```python
from build123d import *

# Parameters (mm, degrees)
F1_DEPTH = 38.1
F2_SIZE  = 8.763


with BuildPart() as f1:
    # F0 (on Front) → F1 (new body)
    with BuildSketch(Plane.XZ):
        Polygon((-6.977107, 9.66563), (-12.7, 0), (-8.651809, -10.447565), (4.802615, -10.447565), (10.988482, 0), (7.243273, 9.66563), align=None)
    extrude(amount=F1_DEPTH)

    # F2
    f2_edges = [f1.edges().sort_by_distance(p)[0] for p in [
        (0.133083, 0, 9.66563),
        (-9.838553, 0, 4.832815),
        (-10.675905, 0, -5.223783),
        (-1.924597, 0, -10.447565),
        (7.895549, 0, -5.223783),
        (9.115878, 0, 4.832815),
    ]]
    chamfer(f2_edges, length=F2_SIZE)


solid = f1.part
```
The listing builds one solid part. Answer for the finished solid, in the listing's coordinates (mm). Coordinates: 2 decimals unless noted, no trailing zeros. Write each loop counter-clockwise with the first axis right and the second up, starting at its lowest first coordinate (ties: lowest second). Pieces come first, ordered by that corner, then holes.
Q1. Section A-A, the plane y = -24 is taken. Write down the section's boundary in (x, z).
Returned:
outline: (-12.7, 0) - (-8.65, -10.45) - (4.8, -10.45) - (10.99, 0) - (7.24, 9.67) - (-6.98, 9.67) - close
Q2. Section D-D, the plane x = -6 is taken. Write down the section's boundary in (y, z), then the cut area to 3 significant figures.
Returned:
outline: (-38.1, -10.45) - (-8.76, -10.45) - (-4.89, -6.58) - (-2.72, -0.55) - (-7.05, 7.95) - (-8.76, 9.67) - (-38.1, 9.67) - close
area: 662 mm2
Q3. Find the intervals of material crossed by line 1 along X through (y, z) = (-8.5, 4.5); line 2 along X through (y, z) = (-28, -6.25); line 3 along Y through (x, z) = (-8.5, -8.5), in increasing order.
Returned:
line 1: x = -9.73 to 8.96
line 2: x = -10.28 to 7.29
line 3: y = -38.1 to -7.92
Q4. Section B-B, the plane x = 0.5 is taken. Write down the section's boundary in (y, z), then the cut area to 3 significant figures.
Returned:
outline: (-38.1, -10.45) - (-8.76, -10.45) - (-1.22, -2.9) - (0, -0.51) - (0, 0.9) - (-8.76, 9.67) - (-38.1, 9.67) - close
area: 689 mm2
Q5. Section C-C, the plane z = -5 is taken. Write down the section's boundary in (x, y).
Returned:
outline: (-10.76, -38.1) - (8.03, -38.1) - (8.03, -8.76) - (1.7, -3.32) - (-4.92, -3.32) - (-10.76, -8.76) - close
Q6. Given P1, Ø6, axis at y = -32, z = 0.5, coming from the +X side; P2, Ø4, axis at y = -28.5, z = -2.5, coming from the -X side; P3, Ø12, axis at y = -13.5, z = 7, coming from the +X side, each flat-ended and moving along its own axis, determine where each tip first touches the part or whether it passes through.
Returned:
P1: stops at x = 10.99
P2: stops at x = -12.51
P3: stops at x = 10.6
